from build123d import *

# Parameters (mm, degrees)
SKETCH1_W              = 54
SKETCH1_H              = 39.25
BOSS_EXTRUDE1_DEPTH    = 46.5
FILLET1_R              = 2
FILLET2_R              = 2
Z_95_START             = -0.023652431
Z_95_BLANK_DEPTH       = 10
Z_95_START_2           = -5.023652431
Z_95_BLANK_2_OUTLINE_R = 2.5
Z_95_BLANK_2_DEPTH     = 5
BODY_MOVE_COPY3_ANGLE  = 180
BODY_MOVE_COPY4_ANGLE  = 89.5
SKETCH4_W              = 54
SKETCH4_H              = 39.25
CUT_EXTRUDE1_DEPTH     = 31
CUT_EXTRUDE2_DEPTH     = 31
BOSS_EXTRUDE2_DEPTH    = 2
FILLET3_R              = 2
FILLET4_R              = 2
FILLET5_R              = 2
FILLET6_R              = 2
SKETCH7_R              = 4.5
CUT_EXTRUDE3_DEPTH     = 3.5


with BuildPart() as part:
    # Sketch1 → Boss-Extrude1 (new body)
    with BuildSketch(Plane(origin=(0, 0, 0), x_dir=(1, 0, 0), z_dir=(0, 1, 0))):
        with Locations((27, 19.625)):
            Rectangle(SKETCH1_W, SKETCH1_H)
    extrude(amount=BOSS_EXTRUDE1_DEPTH)

    # Fillet1
    fillet1_edges = [part.edges().sort_by_distance(p)[0] for p in [
        (0, 23.25, 0),
    ]]
    fillet(fillet1_edges, radius=FILLET1_R)

    # Fillet2
    fillet2_edges = [part.edges().sort_by_distance(p)[0] for p in [
        (0, 23.25, -39.25),
        (54, 23.25, -39.25),
        (54, 23.25, 0),
    ]]
    fillet(fillet2_edges, radius=FILLET2_R)


with BuildPart() as body_2:
    # Z-95 Blank: read off the stored shape, not the designer's step
    # Z-95 Blank outline → Z-95 Blank (new body)
    with BuildSketch(Plane(origin=(0, 0, 0), x_dir=(1, 0, 0), z_dir=(0, 1, 0)).offset(Z_95_START)):
        Polygon((-39.475833264, 51.689675598), (-39.475833264, 48.062948495), (-51.475833264, 46.678320586), (-51.475833264, 23.139646129), (-47.225833264, 23.139646129), (-47.225833264, 35.139646129), (-37.225833264, 35.139646129), (-35.725833264, 5.689675598), (-31.225833264, 5.689675598), (-29.725833264, 35.139646129), (-19.725833264, 35.139646129), (-19.725833264, 23.139646129), (-15.475833264, 23.139646129), (-15.475833264, 46.678320586), (-27.475833264, 48.062948495), (-27.475833264, 51.689675598), align=None)
    extrude(amount=Z_95_BLANK_DEPTH)

    # Z-95 Blank 2 outline → Z-95 Blank 2 (add)
    with BuildSketch(Plane(origin=(0, 0, 0), x_dir=(1, 0, 0), z_dir=(0, 1, 0)).offset(Z_95_START_2)):
        with Locations((-33.475833264, 34.343753809)):
            Circle(Z_95_BLANK_2_OUTLINE_R)
    extrude(amount=Z_95_BLANK_2_DEPTH)


with BuildPart() as body_2_1:
    # Body-Move/Copy3: moved
    add(body_2.part.rotate(Axis((0, 2.476347569, -28.689675598), (1, 0, 0)), BODY_MOVE_COPY3_ANGLE))


with BuildPart() as body_2_2:
    # Body-Move/Copy4: moved
    add(body_2_1.part.rotate(Axis((-33.475833264, 0, -28.689675598), (0, -1, 0)), BODY_MOVE_COPY4_ANGLE))


with BuildPart() as body_2_3:
    # Body-Move/Copy5: moved
    add(body_2_2.part.moved(Location((61.536777905, 5.06338101, 8.948981511))))


with BuildPart() as body_2_4:
    # Body-Move/Copy6: moved
    add(body_2_3.part.moved(Location((0, -0.229742035, 0))))


with BuildPart() as part_1:
    add(part.part)

    # Intersect1: read off the stored shape, not the designer's step
    # Intersect1: cut body 2
    add(body_2_4.part, mode=Mode.SUBTRACT)

    # Sketch4 → Cut-Extrude1 (cut)
    with BuildSketch(Plane(origin=(0, 46.5, 0), x_dir=(1, 0, 0), z_dir=(0, 1, 0))):
        with Locations((27, 19.625)):
            Rectangle(SKETCH4_W, SKETCH4_H)
    extrude(amount=-CUT_EXTRUDE1_DEPTH, mode=Mode.SUBTRACT)

    # Sketch5 → Cut-Extrude2 (cut)
    with BuildSketch(Plane(origin=(0, 0, 0), x_dir=(-1, 0, 0), z_dir=(0, -1, 0))):
        Polygon((-23.713680343, 7.952308665), (-23.713680343, 14.054528407), (-52, 15.742860627), (-52, 2), (-35.766082295, 2), (-35.766082295, 7.952308665), align=None)
        Polygon((-23.713680343, 25.345964802), (-23.713680343, 31.453203507), (-35.766082295, 31.453203507), (-35.766082295, 37.25), (-52, 37.25), (-52, 24.152615413), align=None)
        Polygon((-6.871546498, 12.395456139), (-8.594812047, 2), (-2, 2), (-2, 37.25), (-7.869100925, 37.25), (-6.622123507, 27.553904956), (-3.057950712, 27.553904956), (-3.057950712, 12.395456139), align=None)
    extrude(amount=-CUT_EXTRUDE2_DEPTH, mode=Mode.SUBTRACT)

    # Sketch6 → Boss-Extrude2 (add)
    with BuildSketch(Plane.XZ):
        Polygon((52, -24.152615413), (23.713680343, -25.345964802), (23.713680343, -31.453203507), (35.766082295, -31.453203507), (35.766082295, -37.25), (52, -37.25), align=None)
        Polygon((52, -15.742860627), (23.713680343, -14.054528407), (23.713680343, -7.952308665), (35.766082295, -7.952308665), (35.766082295, -2), (52, -2), align=None)
        Polygon((8.594812047, -2), (6.871546498, -12.395456139), (3.057950712, -12.395456139), (3.057950712, -27.553904956), (6.622123507, -27.553904956), (7.869100925, -37.25), (2, -37.25), (2, -2), align=None)
    extrude(amount=-BOSS_EXTRUDE2_DEPTH)

    # Fillet3
    fillet3_edges = [part_1.edges().sort_by_distance(p)[0] for p in [
        (52, 8.75, -2),
    ]]
    fillet(fillet3_edges, radius=FILLET3_R)

    # Fillet4
    fillet4_edges = [part_1.edges().sort_by_distance(p)[0] for p in [
        (2, 8.75, -2),
    ]]
    fillet(fillet4_edges, radius=FILLET4_R)

    # Fillet5
    fillet5_edges = [part_1.edges().sort_by_distance(p)[0] for p in [
        (52, 8.75, -37.25),
    ]]
    fillet(fillet5_edges, radius=FILLET5_R)

    # Fillet6
    fillet6_edges = [part_1.edges().sort_by_distance(p)[0] for p in [
        (2, 8.75, -37.25),
    ]]
    fillet(fillet6_edges, radius=FILLET6_R)

    # Sketch7 → Cut-Extrude3 (cut)
    with BuildSketch(Plane(origin=(0, 15.5, 0), x_dir=(1, 0, 0), z_dir=(0, 1, 0))):
        Polygon((7.869100925, 37.25), (35.766082295, 37.25), (35.766082295, 31.453203507), (23.713680343, 31.453203507), (23.713680343, 25.345964802), (52, 24.152615413), (52, 15.742860627), (23.713680343, 14.054528407), (23.713680343, 7.952308665), (35.766082295, 7.952308665), (35.766082295, 2), (8.594812047, 2), (6.871546498, 12.395456139), (3.057950712, 12.395456139), (3.057950712, 27.553904956), (6.622123507, 27.553904956), align=None)
        with Locations(Location((22.40708172, 19.691353573, 0), (0, 0, 270))):
            Circle(SKETCH7_R, mode=Mode.SUBTRACT)
    extrude(amount=-CUT_EXTRUDE3_DEPTH, mode=Mode.SUBTRACT)


solid = part_1.part
Design review of the part built by this model. Coordinates are the model's own, in mm. A direction names the side the tool comes from. Round coordinates to 2 decimals unless told otherwise and drop trailing zeros. Loops run counter-clockwise (first coordinate to the right, second up) from the corner with the lowest first, then second, coordinate; pieces in that order, holes last. Notation, with made-up numbers: M -2.5,28 L 29.5,28 A13 cw 29.5,36 Z; hole C -8,-32.5 d7. An arc over 180 degrees is marked long. Answer as a JSON object with one key per item and string values.
Item 1: We need section D-D on x = 35. Give the boundary of the cut face in (y, z), and give its area (3 significant figures).
Answer sheet:
{"outline": "M 0,-39.25 L 15.5,-39.25 L 15.5,-37.25 L 12,-37.25 L 12,-31.45 L 2,-31.45 L 2,-24.87 L 12,-24.87 L 12,-14.73 L 2,-14.73 L 2,-7.95 L 12,-7.95 L 12,-2 L 15.5,-2 L 15.5,0 L 0,0 L 0,-16.73 L 9.81,-16.73 L 9.81,-22.87 L 0,-22.87 Z", "area": "291 mm^2"}
Item 2: Clearance check with flat-ended pins moving along their axes: P1, Ø14.5, axis at x = 43.5, z = -28.5, coming from the +Y side; P2, Ø5.5, axis at x = 23, z = -20, coming from the -Y side; P3, Ø4, axis at x = 39, z = -9.5, coming from the +Y side. State where each tip first meets the part, or that it passes through.
Answer sheet:
{"P1": "stops at y = 12", "P2": "stops at y = 9.81", "P3": "stops at y = 2"}
Item 3: Machinability: for faces 1 (the flat face through (22, 14.81, -20)), 2 (the flat face through (54, 8, -19)), 3 (the flat face through (37.659, 6.93, -14.887)), which of the approach directions +Z, -Z, +X, -X, +Y, -Y give a long, thin tool a straight path to every point of the face, cutting with its end or side? Answer none if there is none.
Answer sheet:
{"face 1": "-Y", "face 2": "+Z, -Z, +X, +Y, -Y", "face 3": "+Y"}
Item 4: Wall thickness on L1, parallel to Z at x = 6, y = 5; L2, parallel to Z at x = 47.5, y = 7.25; L3, parallel to X at y = 7.75, z = -36: over which ranges is each line inside the solid? List them lowest first. Write a range as from..to.
Answer sheet:
{"L1": "z = -39.25..-37.25, -27.55..-25.55, -13.55..-12.4, -2..0", "L2": "z = -39.25..-37.25, -24.34..-22.34, -17.48..-15.47, -2..0", "L3": "x = 0..2.15, 7.71..9.75, 33.47..35.77, 51.85..54"}
Item 5: The part is to be moulded in two halves that separate along X. For faces 4 (the flat face through (5, 7, -27.554)), 5 (the flat face through (27, 15.5, -39)), 6 (the cylindrical face through (53.4, 7.86, -38.68)), say which applies: pulls with the +X half, pulls with the -X half, needs draft (parallel to the pull), parting line crosses it, or undercut.
Answer sheet:
{"face 4": "undercut", "face 5": "needs draft", "face 6": "pulls with the +X half"}
Item 6: We need section A-A on z = -32.5. Give the boundary of the cut face in (x, y).
Answer sheet:
{"outline": "M 0,0 L 9.37,0 L 9.37,9.81 L 21.5,9.81 L 21.5,0 L 54,0 L 54,15.5 L 52,15.5 L 52,2 L 35.77,2 L 35.77,12 L 7.26,12 L 7.26,2 L 2,2 L 2,15.5 L 0,15.5 Z"}
Item 7: We need section C-C on x = 20.5. Give the boundary of the cut face in (y, z).
Answer sheet:
{"outline": "M 0,-39.25 L 15.5,-39.25 L 15.5,-37.25 L 12,-37.25 L 12,-23.77 L 15.5,-23.77 L 15.5,-15.62 L 12,-15.62 L 12,-2 L 15.5,-2 L 15.5,0 L 0,0 L 0,-1.67 L 9.81,-1.67 L 9.81,-18.07 L 14.81,-18.07 L 14.81,-21.31 L 9.81,-21.31 L 9.81,-37.68 L 0,-37.68 Z"}
Item 8: We need section B-B on y = 8. State how many separate pieces and enclosed holes the cut face has, and give its area (3 significant figures).
Answer sheet:
{"separate pieces": "1", "enclosed holes": "4", "area": "645 mm^2"}
